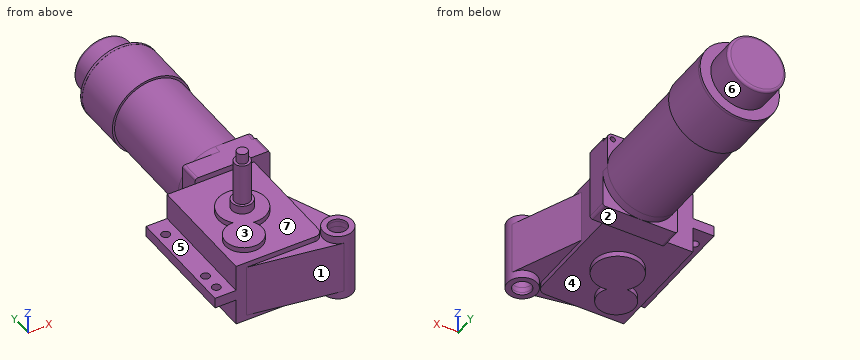
from build123d import *
from build123d.topology import SkipClean

# Parameters (mm, degrees)
SKETCH2_R                   = 47.625
EXTRUDE1_DEPTH              = 63.5
SKETCH3_R                   = 44.958
EXTRUDE2_DEPTH              = 190.5
SKETCH4_R                   = 34.925
EXTRUDE3_DEPTH              = 34.925
FILLET1_R                   = 3.175
SKETCH5_R                   = 3.175
EXTRUDE4_DEPTH              = 9.525
EXTRUDE5_DEPTH              = 25.4
SKETCH7_W                   = 104.775
SKETCH7_H                   = 76.2
EXTRUDE6_DEPTH              = 138.43
EXTRUDE7_DEPTH              = 6.35
EXTRUDE8_START              = -6.35
SKETCH9_R                   = 11.1125
EXTRUDE8_DEPTH              = 63.5
FILLET2_R                   = 9.525
SKETCH10_R                  = 17.78
SKETCH10_R_2                = 11.1125
EXTRUDE9_DEPTH              = 3.175
EXTRUDE9_DIRECTION_2_REACH  = 401.016
SKETCH11_W                  = 25.4
SKETCH11_H                  = 12.7
ATTACHMENT_RAIL_DEPTH       = 138.43
ATTACHMENT_HOLES_DEPTH      = 399.478382273
ATTACHMENT_HOLES_DEPTH_BACK = 399.478382273
SKETCH16_R                  = 5.159375
SKETCH12_R                  = 12.573
EXTRUDE11_DEPTH             = 10.16
SKETCH13_R                  = 9.525
EXTRUDE12_DEPTH             = 50.8
SKETCH14_R                  = 6.35
EXTRUDE13_DEPTH             = 12.7
SKETCH15_R                  = 47.752
EXTRUDE15_DEPTH             = 3.175


with BuildPart() as part:
    # Sketch2 → Extrude1 (new body)
    with BuildSketch(Plane(origin=(0, 0, 0), x_dir=(1, 0, 0), z_dir=(0, 1, 0))):
        with Locations(Location((0, 0, 0), (0, 0, 270))):
            Circle(SKETCH2_R)
    extrude(amount=-EXTRUDE1_DEPTH)

    # Sketch3 → Extrude2 (add)
    with BuildSketch(Plane(origin=(0, 0, 0), x_dir=(1, 0, 0), z_dir=(0, 1, 0))):
        with Locations(Location((0, 0, 0), (0, 0, 270))):
            Circle(SKETCH3_R)
    extrude(amount=-EXTRUDE2_DEPTH)

    # Sketch4 → Extrude3 (add)
    with BuildSketch(Plane(origin=(0, 0, 0), x_dir=(1, 0, 0), z_dir=(0, 1, 0))):
        with Locations(Location((0, 0, 0), (0, 0, 270))):
            Circle(SKETCH4_R)
    extrude(amount=EXTRUDE3_DEPTH)

    # Fillet1
    fillet1_edges = [part.edges().sort_by_distance(p)[0] for p in [
        (0, 34.925, -34.925),
    ]]
    fillet(fillet1_edges, radius=FILLET1_R)

    # Sketch5 → Extrude4 (add)
    with BuildSketch(Plane.XZ.offset(190.5)):
        with BuildLine():
            Line((0, 44.958), (38.608, 44.958))
            ThreePointArc((38.608, 44.958), (43.098128061, 43.098128061), (44.958, 38.608))
            Line((44.958, 38.608), (44.958, 0))
            ThreePointArc((44.958, 0), (-31.790106669, -31.790106669), (0, 44.958))
        make_face()
        with Locations(Location((38.608, 38.608, 0), (0, 0, 90))):
            Circle(SKETCH5_R, mode=Mode.SUBTRACT)
    extrude(amount=EXTRUDE4_DEPTH)

    # Sketch6 → Extrude5 (add)
    with BuildSketch(Plane.XZ.offset(200.025)):
        with BuildLine():
            Line((-41.783, -44.958), (41.783, -44.958))
            ThreePointArc((41.783, -44.958), (44.02806403, -44.02806403), (44.958, -41.783))
            Line((44.958, -41.783), (44.958, 41.783))
            ThreePointArc((44.958, 41.783), (44.02806403, 44.02806403), (41.783, 44.958))
            Line((41.783, 44.958), (-41.783, 44.958))
            ThreePointArc((-41.783, 44.958), (-44.02806403, 44.02806403), (-44.958, 41.783))
            Line((-44.958, 41.783), (-44.958, -41.783))
            ThreePointArc((-44.958, -41.783), (-44.02806403, -44.02806403), (-41.783, -44.958))
        make_face()
    extrude(amount=EXTRUDE5_DEPTH)

    # Sketch7 → Extrude6 (add)
    with BuildSketch(Plane.XZ.offset(225.425)):
        with Locations((-26.4795, 0)):
            Rectangle(SKETCH7_W, SKETCH7_H)
    extrude(amount=EXTRUDE6_DEPTH)

    # Sketch8 → Extrude7 (add)
    with BuildSketch(Plane.XY.offset(38.1)):
        with BuildLine():
            ThreePointArc((-48.596974265, -307.017759799), (-59.433810345, -348.70612023), (-29.96966545, -317.286053756))
            ThreePointArc((-29.96966545, -317.286053756), (-12.684672414, -263.90034502), (-48.596974265, -307.017759799))
        make_face()
    extrude7 = extrude(amount=EXTRUDE7_DEPTH)

    # Mirror1: Extrude7 across plane
    add(extrude7.mirror(Plane.XY))

    # Sketch9 → Extrude8 (add)
    with BuildSketch(Plane.XY.offset(38.1).offset(EXTRUDE8_START)):
        with BuildLine():
            Line((60.100307692, -357.016538462), (25.908, -274.955))
            Line((25.908, -274.955), (25.908, -363.855))
            Line((25.908, -363.855), (-66.167, -363.855))
            Line((-66.167, -363.855), (40.810312139, -381.400578149))
            ThreePointArc((40.810312139, -381.400578149), (57.632240078, -374.886163522), (60.100307692, -357.016538462))
        make_face()
        with Locations((43.688, -363.855)):
            Circle(SKETCH9_R, mode=Mode.SUBTRACT)
    extrude(amount=-EXTRUDE8_DEPTH)

    # Fillet2
    fillet2_edges = [part.edges().sort_by_distance(p)[0] for p in [
        (25.908, -363.855, -34.925),
        (25.908, -363.855, 34.925),
    ]]
    fillet(fillet2_edges, radius=FILLET2_R)

    # Sketch10 → Extrude9 (add)
    with BuildSketch(Plane.XY.offset(38.1)):
        with Locations((43.688, -363.855)):
            Circle(SKETCH10_R)
        with Locations((43.688, -363.855)):
            Circle(SKETCH10_R_2, mode=Mode.SUBTRACT)
    extrude9 = extrude(amount=EXTRUDE9_DEPTH)

    # Sketch10 → Extrude9 direction 2 (add, up to next)
    with BuildSketch(Plane.XY.offset(38.1), mode=Mode.PRIVATE) as extrude9_direction_2_sk1:
        with Locations((43.688, -363.855)):
            Circle(SKETCH10_R)
        with Locations((43.688, -363.855)):
            Circle(SKETCH10_R_2, mode=Mode.SUBTRACT)
    extrude9_direction_2_tool1 = extrude(extrude9_direction_2_sk1.sketch, amount=-EXTRUDE9_DIRECTION_2_REACH, mode=Mode.PRIVATE) - part.part
    extrude9_direction_2 = extrude9_direction_2_tool1.solids().sort_by_distance((26.410894, -363.855, 38.1))[0]
    add(extrude9_direction_2)

    # Mirror2: Extrude9, Extrude9 direction 2 across plane
    with SkipClean():  # the faces are left unmerged after this step: merging them gives an invalid solid
        add(extrude9.mirror(Plane.XY))
        add(extrude9_direction_2.mirror(Plane.XY))

    # Sketch11 → Attachment rail (add)
    with SkipClean():  # the faces are left unmerged after this step: merging them gives an invalid solid
        with BuildSketch(Plane(origin=(0, -225.425, 0), x_dir=(1, 0, 0), z_dir=(0, 1, 0))):
            with Locations((-91.567, 0)):
                Rectangle(SKETCH11_W, SKETCH11_H)
        extrude(amount=-ATTACHMENT_RAIL_DEPTH)

    # Sketch16 → Attachment holes (cut, two sides: drawn at the far end of the back side and taken through both)
    with SkipClean():  # the faces are left unmerged after this step: merging them gives an invalid solid
        with BuildSketch(Plane.XY.offset(-ATTACHMENT_HOLES_DEPTH_BACK)):
            with Locations((-93.63075, -247.17375)):
                Circle(SKETCH16_R)
            with Locations((-93.63075, -327.2282)):
                Circle(SKETCH16_R)
            with Locations((-93.63075, -348.77375)):
                Circle(SKETCH16_R)
        extrude(amount=ATTACHMENT_HOLES_DEPTH + ATTACHMENT_HOLES_DEPTH_BACK, mode=Mode.SUBTRACT)

    # Sketch12 → Extrude11 (add)
    with SkipClean():  # the faces are left unmerged after this step: merging them gives an invalid solid
        with BuildSketch(Plane.XY.offset(44.45)):
            with Locations((-26.4795, -288.925)):
                Circle(SKETCH12_R)
        extrude(amount=EXTRUDE11_DEPTH)

    # Sketch13 → Extrude12 (add)
    with SkipClean():  # the faces are left unmerged after this step: merging them gives an invalid solid
        with BuildSketch(Plane.XY.offset(54.61)):
            with Locations((-26.4795, -288.925)):
                Circle(SKETCH13_R)
        extrude(amount=EXTRUDE12_DEPTH)

    # Sketch14 → Extrude13 (add)
    with SkipClean():  # the faces are left unmerged after this step: merging them gives an invalid solid
        with BuildSketch(Plane.XY.offset(105.41)):
            with Locations((-26.4795, -288.925)):
                Circle(SKETCH14_R)
        extrude(amount=EXTRUDE13_DEPTH)

    # Sketch15 → Extrude15 (add)
    with SkipClean():  # the faces are left unmerged after this step: merging them gives an invalid solid
        with BuildSketch(Plane(origin=(0, 0, 0), x_dir=(1, 0, 0), z_dir=(0, 1, 0))):
            with Locations(Location((0, 0, 0), (0, 0, 270))):
                Circle(SKETCH15_R)
        extrude(amount=-EXTRUDE15_DEPTH)


solid = part.part
For this review, take the finished solid that the model builds, in its own axes (mm). Face numbers are marked on the shaded views. A direction names the side the tool comes from. Round coordinates to 2 decimals unless told otherwise and drop trailing zeros. Order: outer loops, then holes, each group sorted by start corner. A loop starts at its lowest first (then second) coordinate and runs counter-clockwise, first axis right, second up. Notation, with made-up numbers: (57.5, -8) -> (69.5, -8) arc R24 ccw to (69.5, 17) -> close; hole circle Ø3 at (12.25, -11.5). An arc over 180 degrees is marked (long way). Write item = value, one per line. Start each with the question number.
1) The part is to be moulded in two halves that separate along Y. For the marked faces 1, 2 and 3, say which applies: +Y half, -Y half, draft (parallel to the pull), parting line (faces both ways), or undercut.
2) Take a section at C-C on y = -105.5. State the section outline as (x, z) points, plus the area to 3 significant figures.
3) Insertion check: pin 1 (12 mm diameter, centred on x = 2, y = -236.5, fed in from -Z); pin 2 (10.5 mm diameter, centred on y = -216, z = -3.5, fed in from +X); pin 3 (3 mm diameter, centred on y = -106, z = 29.5, fed in from +X). Each pin has a flat end and moves straight along its axis. Give the tip position at first contact, or say it passes through.
4) Take a section at B-B on x = -61.5. State the section outline as (y, z) points (3 decimals), plus the area to 3 significant figures.
5) Tool access review of the marked faces 4, 5, 6 and 7: name each direction out of +Z, -Z, +X, -X, +Y, -Y from which nothing blocks a thin tool from reaching the whole face with its end or side.
6) Take a section at A-A on y = -232. State the section outline as (x, z) points.
7) To check wall thickness, follow line 1 (Z direction, x = -28, y = -272.5); line 2 (Y direction, x = -15.5, z = 37) (3 decimals). State the ranges of each line that lie inside material, in increasing order. Write a range as from..to.
8) Take a section at D-D on y = -41. State the section outline as (x, z) points (3 decimals), plus the area to 3 significant figures.
Verdict:
q1.face_1 = -Y half
q1.face_2 = draft
q1.face_3 = undercut
q2.outline = circle Ø89.92 at (0, 0)
q2.area = 6,350 mm2
q3.pin_1 = -38.1
q3.pin_2 = 44.96
q3.pin_3 = 35.17
q4.outline = (-364.62, -31.75) -> (-363.855, -31.75) -> (-363.855, -38.1) -> (-347.415, -38.1) -> (-347.415, -44.45) -> (-311.07, -44.45) -> (-311.07, -38.1) -> (-225.425, -38.1) -> (-225.425, 38.1) -> (-311.07, 38.1) -> (-311.07, 44.45) -> (-347.415, 44.45) -> (-347.415, 38.1) -> (-363.855, 38.1) -> (-363.855, 31.75) -> (-364.62, 31.75) -> close
q4.area = 11,100 mm2
q5.face_4 = -Z
q5.face_5 = +Z, -X, +Y, -Y
q5.face_6 = +Y
q5.face_7 = +Z
q6.outline = (-104.27, -6.35) -> (-78.87, -6.35) -> (-78.87, -38.1) -> (25.91, -38.1) -> (25.91, 38.1) -> (-78.87, 38.1) -> (-78.87, 6.35) -> (-104.27, 6.35) -> close
q7.line_1 = -44.45..44.45
q7.line_2 = -363.855..0
q8.outline = circle Ø95.25 at (0, 0)
q8.area = 7,130 mm2
